Autodesk Inventor part; units mm, degrees
ref_plane "YZ Plane" through (0, 0, 0) normal (1, 0, 0) x (0, 1, 0)
ref_plane "XZ Plane" through (0, 0, 0) normal (0, 1, 0) x (-1, 0, 0)
ref_plane "XY Plane" through (0, 0, 0) normal (0, 0, 1) x (1, 0, 0)
sketch "Skizze1" plane through (0, 0, 0) normal (1, 0, 0) x (0, 1, 0)
  line L0 (0, -29.1045) -> (0, 0)
  line L1 (0, 0) -> (0, -20.5338)
  line L2 (0, 0) -> (34.35, 0)
  line L3 (34.35, 0) -> (34.35, -15)
  line L4 (34.35, -15) -> (38.05, -15)
  line L5 (38.05, -15) -> (38.05, -25)
  line L6 (38.05, -25) -> (10, -25)
  line L7 (10, -25) -> (10, -110)
  line L8 (10, -110) -> (0, -110)
  line L9 (0, 0) -> (0, -24.283)
  line L10 (34.35, 0) -> (0, 0)
  line L11 (0, -132) -> (0, 22)
  line L12 (0, -110) -> (0, 0)
  dimension "d0" = 15
  dimension "d1" = 25
  dimension "d2" = 76.1
  dimension "d3" = 68.7
  dimension "d4" = 20
  dimension "d6" = 85
revolve "Umdrehung1" add sketch "Skizze1" angle 360 about axis through (0, 0, -110) along (0, 0, 1)
thread "Gewinde1"
chamfer "Fase1" distance 2 angle 45 1 edges at (0, -10, -110)
properties part number "Rad Aufnahme" material "Stahl"
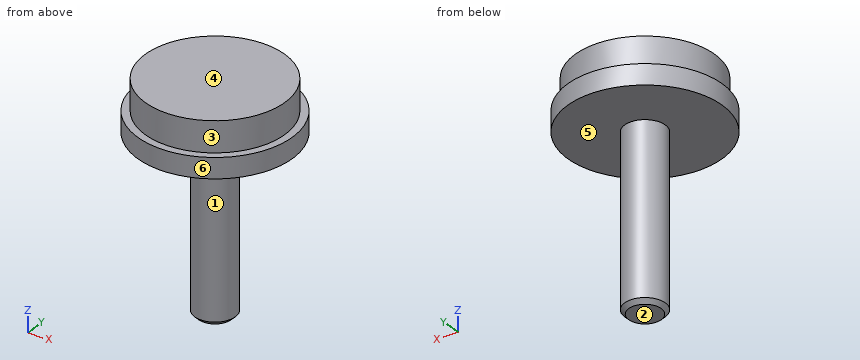
Design review of the part built by this model. Coordinates are the model's own, in mm. Face numbers are marked on the shaded views. A direction names the side the tool comes from. Coordinates: 2 decimals unless noted, no trailing zeros. Order: outer loops, then holes, each group sorted by start corner. A loop starts at its lowest first (then second) coordinate and runs counter-clockwise, first axis right, second up. Notation, with made-up numbers: (3.5, -35) -> (39.5, -35) arc R28 ccw to (39.5, -9) -> close; hole circle Ø8 at (66, -9). An arc over 180 degrees is marked (long way). Use one line per item in the form item = value. Start each with the question number.
(1) Add section D-D on y = -25.5. State the section outline as (x, z) points, plus the area to 3 significant figures.
(2) For probe 1 along Z at (x, y) = (-20, -2); probe 2 along Z at (x, y) = (23.5, -29); probe 3 along Y at (x, z) = (-30.5, -14.5), list the stretches that pass through material, from the lowest coordinate up.
(3) Add section C-C on z = -12. State the section outline as (x, y) points.
(4) Add section A-A on y = 0. State the section outline as (x, z) points.
(5) Insertion check: pin 1 (2 mm diameter, centred on x = -9.5, z = -61, fed in from -Y); pin 2 (12 mm diameter, centred on x = -21, y = 15.5, fed in from -Z); pin 3 (12 mm diameter, centred on y = -13, z = -36.5, fed in from +X). Each pin has a flat end and moves straight along its axis. Give the tip position at first contact, or say it passes through.
(6) The part is to be moulded in two halves that separate along Z. For the marked faces 4, 5 and 6, say which applies: +Z half, -Z half, draft (parallel to the pull), parting line (faces both ways), or undercut.
(7) For the marked faces 1, 2 and 3, list the 3-axis set-ups (+Z, -Z, +X, -X, +Y, -Y) from which the entire face can be reached by the end or side of a thin tool; tool diameter is ignored.
Answer block:
q1.outline = (-28.24, -25) -> (28.24, -25) -> (28.24, -15) -> (23.01, -15) -> (23.01, 0) -> (-23.01, 0) -> (-23.01, -15) -> (-28.24, -15) -> close
q1.area = 1,260 mm²
q2.probe_1 = -25 to 0
q2.probe_2 = -25 to -15
q2.probe_3 = -15.8 to 15.8
q3.outline = circle Ø68.7 at (0, 0)
q4.outline = (-38.05, -25) -> (-10, -25) -> (-10, -108) -> (-8, -110) -> (8, -110) -> (10, -108) -> (10, -25) -> (38.05, -25) -> (38.05, -15) -> (34.35, -15) -> (34.35, 0) -> (-34.35, 0) -> (-34.35, -15) -> (-38.05, -15) -> close
q5.pin_1 = -5.27
q5.pin_2 = -25
q5.pin_3 = 7.14
q6.face_4 = +Z half
q6.face_5 = -Z half
q6.face_6 = draft
q7.face_1 = -Z
q7.face_2 = -Z, +X, -X, +Y, -Y
q7.face_3 = +Z
